```python
from build123d import *

# Parameters (mm, degrees)
F3_D     = 8
F3_DEPTH = 15
F3_TIP   = 2.4034424761
F4_W     = 3
F4_H     = 21
F5_DEPTH = 12.5


with BuildPart() as f1:
    # F0 (on Right) → F1 (revolve)
    with BuildSketch(Plane.YZ):
        Polygon((-61.5567314936, 4.5), (-61.5567314936, 0), (229.4432685064, 0), (229.4432685064, 37.5), (-7.5567314936, 37.5), (-7.5567314936, 21.5), (-25.5567314936, 21.5), (-31.5567314936, 15.5), (-31.5567314936, 10.75), (-40.0567314936, 10.75), (-40.0567314936, 9), (-43.5567314936, 9), (-43.5567314936, 10.5), (-55.5567314936, 10.5), align=None)
    revolve(axis=Axis((0, 83.9432685064, 0), (0, 1, 0)))

    # F3
    with Locations(Plane.XZ.offset(61.5567314936)):
        with Locations((0, 0)):
            Hole(F3_D / 2, depth=F3_DEPTH)
            with Locations((0, 0, -(F3_DEPTH + F3_TIP / 2))):  # 118° drill point
                Cone(0, F3_D / 2, F3_TIP, mode=Mode.SUBTRACT)

    # F4 (on Top) → F5 (cut, symmetric)
    with BuildSketch(Plane.XY):
        with Locations((11, -42.0567314936)):
            Rectangle(F4_W, F4_H)
        with Locations((-11, -42.0567314936)):
            Rectangle(F4_W, F4_H)
    extrude(amount=F5_DEPTH, both=True, mode=Mode.SUBTRACT)


solid = f1.part
```
Work out the finished part from the listing and answer in its coordinate system (mm). A direction names the side the tool comes from. Round coordinates to 2 decimals unless told otherwise and drop trailing zeros. Loops run counter-clockwise (first coordinate to the right, second up) from the corner with the lowest first, then second, coordinate; pieces in that order, holes last. Notation, with made-up numbers: M 17.25,83 L 76.25,83 A12 ccw 76.25,95 Z; hole C -36,3 d3. An arc over 180 degrees is marked long. Use CSV: the item, a comma, the result in double quotes.
Q1. Section C-C, the plane y = 66.5 is taken. Determine the outline of the cut face in (x, z).
Determined:
outline,"C 0,0 d75"
Q2. A tool of negligible diameter and unlimited length cuts with its end or side. For faces 1 (the flat face through (1, 229.443, 1)), 2 (the flat face through (-16, -7.557, 16)), 3 (the flat face through (9.5, -36, 0)), 4 (the flat face through (-8, -40.057, -5)), 5 (the flat face through (-9.5, -36, 0)), from which of +Z, -Z, +X, -X, +Y, -Y can it reach the whole face along a straight path? Write none if from no direction.
Determined:
face 1,"+Z, -Z, +X, -X, +Y"
face 2,"-Y"
face 3,"+Z, -Z, +X"
face 4,"none"
face 5,"+Z, -Z, -X"
Q3. Section B-B, the plane x = 29 is taken. Determine the outline of the cut face in (y, z), then the cut area to 3 significant figures.
Determined:
outline,"M -7.56,-23.77 L 229.44,-23.77 L 229.44,23.77 L -7.56,23.77 Z"
area,"11,300 mm2"
Q4. Consider L1, parallel to Z at x = 0, y = -55.25; L2, parallel to X at y = -50, z = 0; L3, parallel to Y at x = -29, z = -20.5. Determine where each line is inside the solid, lowest interval first.
Determined:
L1,"-10.5 to -4, 4 to 10.5"
L2,"-9.5 to -4, 4 to 9.5"
L3,"-7.56 to 229.44"
Q5. The mould has two halves that part along Z. Classify faces 6 (the cylindrical face through (0.867, -53.952, -3.905)), 7 (the cylindrical face through (0.16, -35.87, -10.75)), 8 (the conical face through (1.439, -61.265, 4.57)): pulls with the +Z half, pulls with the -Z half, needs draft (parallel to the pull), parting line crosses it, or undercut.
Determined:
face 6,"undercut"
face 7,"pulls with the -Z half"
face 8,"parting line crosses it"
Q6. Section A-A, the plane y = -18 is taken. Determine the outline of the cut face in (x, z).
Determined:
outline,"C 0,0 d43"
Q7. Each of these flat-tipped pins is pushed along its axis until it touches: pin 1 (2.5 mm diameter, centred on y = -37, z = -0.5, fed in from -X); pin 2 (1 mm diameter, centred on x = 22, y = 143, fed in from -Z); pin 3 (6 mm diameter, centred on y = 111.5, z = 24.5, fed in from -X). Where does it stop, or does it pass through?
Determined:
pin 1,"x = -9.5"
pin 2,"z = -30.72"
pin 3,"x = -30.72"
